```python
from build123d import *

# Parameters (mm, degrees)
EXTRUDE_2_DEPTH     = 14
FILLET_1_RADIUS     = 7
FILLET_1_LENGTH     = 6.553419282
FILLET_2_RADIUS     = 7
FILLET_2_LENGTH     = 6.553419282
EXTRUDE_3_DEPTH     = 14
FILLET_3_RADIUS     = 7
FILLET_3_LENGTH     = 6
FILLET_4_RADIUS     = 7
FILLET_4_LENGTH     = 6
EXTRUDE_5_REACH     = 125.088
SKETCH_8_R          = 2.45
SKETCH_8_W          = 10.538484084
SKETCH_8_H          = 14
EXTRUDE_6_REACH     = 124.55
SKETCH_11_R         = 2.425
SKETCH_13_W         = 25.960961566
SKETCH_13_H         = 14
EXTRUDE_7_DEPTH     = 11
CUT_EXTRUDE_2_REACH = 137.882
SKETCH_14_R         = 5
FILLET_5_R          = 1


with BuildPart() as part:
    # Sketch 1 → Extrude 2 (new body)
    with BuildSketch(Plane(origin=(0, 0, 0), x_dir=(1, 0, 0), z_dir=(0, 1, 0))):
        with BuildLine():
            Line((5, 0), (5, 52.718048915))
            ThreePointArc((5, 52.718048915), (4.918829182, 53.989594298), (4.676634468, 55.240497206))
            Line((4.676634468, 55.240497206), (2.323365532, 64.268124597))
            ThreePointArc((2.323365532, 64.268124597), (2.081170818, 65.519027505), (2, 66.790572889))
            Line((2, 66.790572889), (2, 120))
            Line((2, 120), (-4.553419282, 120))
            Line((-4.553419282, 120), (-4.553419282, 66.790572889))
            ThreePointArc((-4.553419282, 66.790572889), (-4.472248464, 65.519027505), (-4.23005375, 64.268124597))
            Line((-4.23005375, 64.268124597), (-1.876784815, 55.240497206))
            ThreePointArc((-1.876784815, 55.240497206), (-1.6345901, 53.989594298), (-1.553419282, 52.718048915))
            Line((-1.553419282, 52.718048915), (-1.553419282, 0))
            Line((-1.553419282, 0), (5, 0))
        make_face()
    extrude(amount=EXTRUDE_2_DEPTH)

    # Fillet 1: full round fillet: the end face becomes a half cylinder, R = half its width
    fillet_1_face = Plane((1.723290359, 7, 0), x_dir=(1, 0, 0), z_dir=(0, 0, 1))  # on the end face: x along it, z out of the body
    fillet_1_slab = fillet_1_face.offset(-FILLET_1_RADIUS / 2) * Box(FILLET_1_LENGTH, 2 * FILLET_1_RADIUS, FILLET_1_RADIUS, mode=Mode.PRIVATE)  # the body's end, R deep
    fillet_1_round = Plane((1.723290359, 7, -7), x_dir=(0, 0, 1), z_dir=(1, 0, 0)) * Cylinder(FILLET_1_RADIUS, FILLET_1_LENGTH, mode=Mode.PRIVATE)  # its axis R under the face
    add(fillet_1_slab - fillet_1_round, mode=Mode.SUBTRACT)

    # Fillet 2: full round fillet: the end face becomes a half cylinder, R = half its width
    fillet_2_face = Plane((-1.276709641, 7, -120), x_dir=(-1, 0, 0), z_dir=(0, 0, -1))  # on the end face: x along it, z out of the body
    fillet_2_slab = fillet_2_face.offset(-FILLET_2_RADIUS / 2) * Box(FILLET_2_LENGTH, 2 * FILLET_2_RADIUS, FILLET_2_RADIUS, mode=Mode.PRIVATE)  # the body's end, R deep
    fillet_2_round = Plane((-1.276709641, 7, -113), x_dir=(0, 0, -1), z_dir=(-1, 0, 0)) * Cylinder(FILLET_2_RADIUS, FILLET_2_LENGTH, mode=Mode.PRIVATE)  # its axis R under the face
    add(fillet_2_slab - fillet_2_round, mode=Mode.SUBTRACT)

    # Sketch 8 → Extrude 5 (add, up to next)
    with BuildSketch(Plane(origin=(-18.553419282, 0, 0), x_dir=(0, 0, -1), z_dir=(1, 0, 0)), mode=Mode.PRIVATE) as extrude_5_sk1:
        with Locations(Location((7, 7, 0), (0, 0, 180))):
            Circle(SKETCH_8_R)
    extrude_5_tool1 = extrude(extrude_5_sk1.sketch, amount=EXTRUDE_5_REACH, mode=Mode.PRIVATE) - part.part
    # Sketch 8 → Extrude 5 (add, up to next)
    with BuildSketch(Plane(origin=(-18.553419282, 0, 0), x_dir=(0, 0, -1), z_dir=(1, 0, 0)), mode=Mode.PRIVATE) as extrude_5_sk2:
        with Locations((47.448806873, 7)):
            Rectangle(SKETCH_8_W, SKETCH_8_H)
    extrude_5_tool2 = extrude(extrude_5_sk2.sketch, amount=EXTRUDE_5_REACH, mode=Mode.PRIVATE) - part.part


with BuildPart() as body_2:
    # Sketch 4 → Extrude 3 (new body)
    with BuildSketch(Plane(origin=(0, 0, 0), x_dir=(1, 0, 0), z_dir=(0, 1, 0))):
        with BuildLine():
            Line((-18.553419282, 0), (-24.553419282, 0))
            Line((-24.553419282, 0), (-24.553419282, 52.718048915))
            ThreePointArc((-24.553419282, 52.718048915), (-24.472248464, 53.989594298), (-24.23005375, 55.240497206))
            Line((-24.23005375, 55.240497206), (-21.876784815, 64.268124597))
            ThreePointArc((-21.876784815, 64.268124597), (-21.6345901, 65.519027505), (-21.553419282, 66.790572889))
            Line((-21.553419282, 66.790572889), (-21.553419282, 120))
            Line((-21.553419282, 120), (-15.553419282, 120))
            Line((-15.553419282, 120), (-15.553419282, 66.790572889))
            ThreePointArc((-15.553419282, 66.790572889), (-15.6345901, 65.519027505), (-15.876784815, 64.268124597))
            Line((-15.876784815, 64.268124597), (-18.23005375, 55.240497206))
            ThreePointArc((-18.23005375, 55.240497206), (-18.472248464, 53.989594298), (-18.553419282, 52.718048915))
            Line((-18.553419282, 52.718048915), (-18.553419282, 0))
        make_face()
    extrude(amount=EXTRUDE_3_DEPTH)

    # Fillet 3: full round fillet: the end face becomes a half cylinder, R = half its width
    fillet_3_face = Plane((-18.553419282, 7, -120), x_dir=(-1, 0, 0), z_dir=(0, 0, -1))  # on the end face: x along it, z out of the body
    fillet_3_slab = fillet_3_face.offset(-FILLET_3_RADIUS / 2) * Box(FILLET_3_LENGTH, 2 * FILLET_3_RADIUS, FILLET_3_RADIUS, mode=Mode.PRIVATE)  # the body's end, R deep
    fillet_3_round = Plane((-18.553419282, 7, -113), x_dir=(0, 0, -1), z_dir=(-1, 0, 0)) * Cylinder(FILLET_3_RADIUS, FILLET_3_LENGTH, mode=Mode.PRIVATE)  # its axis R under the face
    add(fillet_3_slab - fillet_3_round, mode=Mode.SUBTRACT)

    # Fillet 4: full round fillet: the end face becomes a half cylinder, R = half its width
    fillet_4_face = Plane((-21.553419282, 7, 0), x_dir=(1, 0, 0), z_dir=(0, 0, 1))  # on the end face: x along it, z out of the body
    fillet_4_slab = fillet_4_face.offset(-FILLET_4_RADIUS / 2) * Box(FILLET_4_LENGTH, 2 * FILLET_4_RADIUS, FILLET_4_RADIUS, mode=Mode.PRIVATE)  # the body's end, R deep
    fillet_4_round = Plane((-21.553419282, 7, -7), x_dir=(0, 0, 1), z_dir=(1, 0, 0)) * Cylinder(FILLET_4_RADIUS, FILLET_4_LENGTH, mode=Mode.PRIVATE)  # its axis R under the face
    add(fillet_4_slab - fillet_4_round, mode=Mode.SUBTRACT)


with BuildPart() as part_1:
    add(part.part)

    add(body_2.part)  # Extrude 5 merges body 2
    add(extrude_5_tool1.solids().sort_by_distance((-18.553419, 7, -7))[0])
    add(extrude_5_tool2.solids().sort_by_distance((-18.553419, 7, -47.448807))[0])

    # Sketch 11 → Extrude 6 (add, up to next)
    with BuildSketch(Plane(origin=(-15.553419282, 0, 0), x_dir=(0, 0, -1), z_dir=(1, 0, 0)), mode=Mode.PRIVATE) as extrude_6_sk1:
        with Locations(Location((88.803678257, 7, 0), (0, 0, 180))):
            Circle(SKETCH_11_R)
    extrude_6_tool1 = extrude(extrude_6_sk1.sketch, amount=EXTRUDE_6_REACH, mode=Mode.PRIVATE) - part_1.part
    add(extrude_6_tool1.solids().sort_by_distance((-15.553419, 7, -88.803678))[0])

    # Sketch 13 → Extrude 7 (add)
    with BuildSketch(Plane(origin=(-15.553419282, 0, 0), x_dir=(0, 0, -1), z_dir=(1, 0, 0))):
        with Locations((120.606040711, 7)):
            Rectangle(SKETCH_13_W, SKETCH_13_H)
    extrude(amount=EXTRUDE_7_DEPTH)

    # Sketch 14 → Cut-Extrude 2 (cut, up to next)
    with BuildSketch(Plane.ZY.offset(15.553419282), mode=Mode.PRIVATE) as cut_extrude_2_sk1:
        with Locations((-126.442783906, 7)):
            Circle(SKETCH_14_R)
    cut_extrude_2_tool1 = extrude(cut_extrude_2_sk1.sketch, amount=-CUT_EXTRUDE_2_REACH, mode=Mode.PRIVATE) & part_1.part
    add(cut_extrude_2_tool1.solids().sort_by_distance((-15.553419, 7, -126.442784))[0], mode=Mode.SUBTRACT)

    # Fillet 5
    fillet_5_edges = [part_1.edges().sort_by_distance(p)[0] for p in [
        (-10.053419282, 0, -133.586521494),
        (-10.053419282, 14, -133.586521494),
    ]]
    fillet(fillet_5_edges, radius=FILLET_5_R)


solid = part_1.part
```
Here's how the part is built. I have some questions about the finished solid (model axes, mm). A direction names the side the tool comes from. Coordinates: 2 decimals unless noted, no trailing zeros. Order: outer loops, then holes, each group sorted by start corner. A loop starts at its lowest first (then second) coordinate and runs counter-clockwise, first axis right, second up.
1) Imagine slicing it at B-B on x = -12. List the corners of the cut face in (y, z) for me (3 decimals), and give its area (3 significant figures).
2) Imagine slicing it at C-C on y = 7. State how many separate pieces and enclosed holes the cut face has, and give its area (3 significant figures).
3) I need wall thicknesses on line 1 (X direction, y = 7.25, z = -70.5); line 2 (X direction, y = 8.5, z = -39.5); line 3 (X direction, y = 13, z = -108). Which ranges of each line are inside material? Lowest first, please.
4) Imagine slicing it at D-D on z = -109. List the corners of the cut face in (x, y) for me.
5) We'd pull the mould along X, two halves only. Please class faces 1 (the face through (2.083, 6.902, -65.501)), 2 (the face through (-19, 7, -120)), 3 (the face through (-21.637, 6.902, -65.501)), 4 (the face through (-3.07, 6.9, -59.82)): +X half, -X half, draft (parallel to the pull), parting line (faces both ways), or undercut.
6) Which directions (+Z, -Z, +X, -X, +Y, -Y) give clear straight access to the entire face, cutting with the end or side of a thin tool? Please do faces 5 (the face through (-21.553, 7, -93)), 6 (the face through (2, 7, -93)), 7 (the face through (-10.13, 6.893, -91.226)), 8 (the face through (-17.037, 6.902, -59.818)).
7) Imagine slicing it at A-A on z = -11. List the corners of the cut face in (x, y) for me, and give its area (3 significant figures).
8) Will these pins go through, and if not, where does the flat tip stop? pin 1 (7 mm diameter, centred on y = 7.5, z = -84, fed in from -X); pin 2 (1.5 mm diameter, centred on x = -12.5, y = 9.5, fed in from +Z); pin 3 (7 mm diameter, centred on y = 9.5, z = -122.5, fed in from +X).
Response values:
1. outline: (0, -132.587) arc R1 ccw to (1, -133.587) - (13, -133.587) arc R1 ccw to (14, -132.587) - (14, -107.626) - (0, -107.626) - close; (0, -52.718) - (14, -52.718) - (14, -42.18) - (0, -42.18) - close; circle Ø4.9 at (7, -7); circle Ø4.85 at (7, -88.804); hole circle Ø10 at (7, -126.443)
1. area: 469 mm2
2. separate pieces: 2
2. enclosed holes: 3
2. area: 2,000 mm2
3. line 1: x = -21.55 to -15.55, -4.55 to 2
3. line 2: x = -24.55 to -18.55, -1.55 to 5
3. line 3: x = -21.55 to 2
4. outline: (-21.55, 0) - (2, 0) - (2, 14) - (-21.55, 14) - close
5. face 1: +X half
5. face 2: draft
5. face 3: -X half
5. face 4: undercut
6. face 5: -Z, -X, +Y, -Y
6. face 6: -Z, +X, +Y, -Y
6. face 7: none
6. face 8: +Y, -Y
7. outline: (-24.55, 0) - (-18.55, 0) - (-18.55, 14) - (-24.55, 14) - close; (-1.55, 0) - (5, 0) - (5, 14) - (-1.55, 14) - close
7. area: 176 mm2
8. pin 1: stops at x = -21.55
8. pin 2: stops at z = -5.29
8. pin 3: stops at x = 2
